Design review of the part built by this model. Coordinates are the model's own, in mm. Give positions to 0.01 mm unless a question says otherwise; leave off trailing zeros. Loops run counter-clockwise (first coordinate to the right, second up) from the corner with the lowest first, then second, coordinate; pieces in that order, holes last. Notation, with made-up numbers: (50, 85) - (80, 85) arc R14 cw to (80, 111) - close; hole circle Ø11 at (64.25, 17.25). An arc over 180 degrees is marked (long way). Write each question's results on one line, items separated by ' | '.
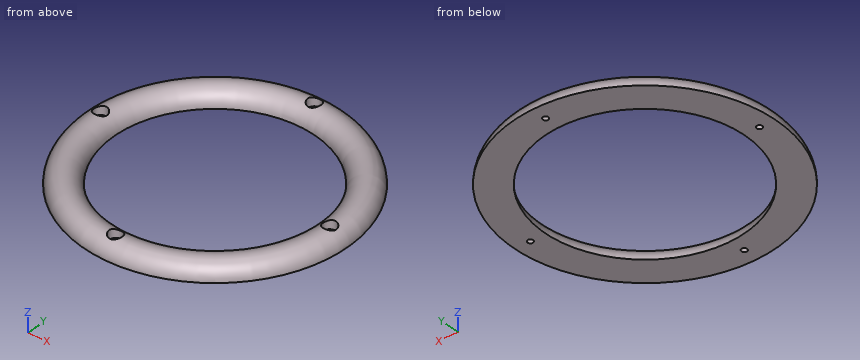
```python
from build123d import *

# Parameters (mm, degrees)
F2_R     = 6
F3_DEPTH = 14
F5_R     = 6
F5_R_2   = 2.5
F6_DEPTH = 6
F7_COUNT = 4


with BuildPart() as f1:
    # F0 (on Front) → F1 (revolve)
    with BuildSketch(Plane.XZ):
        with BuildLine():
            Line((-118, 0), (-90, 0))
            ThreePointArc((-90, 0), (-104, 14), (-118, 0))
        make_face()
    revolve(axis=Axis((0, 0, 34.595653), (0, 0, 1)))

    # F2 (on Top) → F3 (cut)
    with BuildSketch(Plane.XY):
        with Locations((0, -104)):
            Circle(F2_R)
        with Locations((104, 0)):
            Circle(F2_R)
        with Locations((0, 104)):
            Circle(F2_R)
        with Locations((-104, 0)):
            Circle(F2_R)
    extrude(amount=F3_DEPTH, mode=Mode.SUBTRACT)

    # F5 (on offset) → F6 (join)
    with BuildSketch(Plane.XY.offset(6)):
        with Locations((104, 0)):
            Circle(F5_R)
        with Locations((104, 0)):
            Circle(F5_R_2, mode=Mode.SUBTRACT)
    extrude(amount=-F6_DEPTH)

    # F7: F1 ×4 about axis
    f7_axis = Axis((0, 0, 34.595653), (0, 0, 1))


with BuildPart() as f1_1:
    add(f1.part)
    for i in range(1, F7_COUNT):
        add(f1.part.rotate(f7_axis, i * 360 / F7_COUNT))


solid = f1_1.part
```
Item 1: We need section A-A on z = 9. Give the boundary of the cut face in (x, y), then the cut area to 3 significant figures.
Output values:
outline: circle Ø229.45 at (0, 0); hole circle Ø12 at (-104, 0); hole circle Ø186.55 at (0, 0); hole circle Ø12 at (0, -104); hole circle Ø12 at (0, 104); hole circle Ø12 at (104, 0) | area: 13,600 mm²
Item 2: Wall thickness on probe 1 along Y at (x, z) = (-17, 4.75); probe 2 along X at (y, z) = (56, 10.75); probe 3 along Y at (x, z) = (104, 4): over which ranges is each line inside the solid? List them lowest first.
Output values:
probe 1: y = -115.93 to -89.23, 89.23 to 115.93 | probe 2: x = -98.11 to -76.78, 76.78 to 98.11 | probe 3: y = -54.5 to -2.5, 2.5 to 54.5
Item 3: Clearance check with flat-ended pins moving along their axes: P1, Ø1.5, axis at y = 59, z = 2, coming from the -X side; P2, Ø6, axis at x = -106, y = 0.5, coming from the +Z side; P3, Ø4, axis at x = -24.5, z = 6.5, coming from the +Y side. State where each tip first meets the part, or that it passes through.
Output values:
P1: stops at x = -102.47 | P2: stops at z = 6 | P3: stops at y = 114.78
